Check sheet for the modelled part. Datum: model origin and axes. Units: mm. Round coordinates to 2 decimals unless told otherwise and drop trailing zeros. Write each loop counter-clockwise with the first axis right and the second up, starting at its lowest first coordinate (ties: lowest second). Pieces come first, ordered by that corner, then holes. Notation, with made-up numbers: (24.25, 79.5) -> (60.25, 79.5) arc R34 ccw to (60.25, 114.5) -> close; hole circle Ø5 at (60, 9). An arc over 180 degrees is marked (long way). Put each result on its own line as item: value. Start each with the question number.
from build123d import *

# Parameters (mm, degrees)
SKETCH1_R           = 4.7625
BOSS_EXTRUDE1_DEPTH = 4.7625


with BuildPart() as part:
    # Sketch1 → Boss-Extrude1 (new body)
    with BuildSketch(Plane.XY):
        Polygon((0, 0), (0, -45.252735849), (269.24, 127.295542021), (269.24, 172.54827787), align=None)
        with Locations(Location((9.525, -10.651818651, 0), (0, 0, 180))):
            Circle(SKETCH1_R, mode=Mode.SUBTRACT)
        with Locations(Location((28.575, -10.651818651, 0), (0, 0, 180))):
            Circle(SKETCH1_R, mode=Mode.SUBTRACT)
        with Locations(Location((239.234787134, 136.668181349, 0), (0, 0, 180))):
            Circle(SKETCH1_R, mode=Mode.SUBTRACT)
        with Locations(Location((258.284787134, 136.668181349, 0), (0, 0, 180))):
            Circle(SKETCH1_R, mode=Mode.SUBTRACT)
    extrude(amount=BOSS_EXTRUDE1_DEPTH)


solid = part.part
1. Gauge pin test, flat ends, axial feed: P1, Ø11, axis at x = 258.28, y = 136.67, coming from the -Z side; P2, Ø2, axis at y = 44, z = 2, coming from the +X side; P3, Ø1, axis at y = 110, z = 3.5, coming from the -X side. Record the tip position at first contact, or that the pin passes through.
2. Section check C-C, the plane x = 67. Enter the section's corners in (y, z), then the cut area to 3 significant figures.
3. Draft check along Y on faces 1 (the flat face through (136.5, 87.48, 2.35)), 2 (the flat face through (132.735, 39.814, 2.348)), 3 (the cylindrical face through (29.6, -6, 2.3)). Enter one of: released by +Y, released by -Y, zero draft, split by the parting line, or undercut.
4. Section check A-A, the plane z = 1.25. Enter the section's corners in (x, y) (1 decimal), then the cut area to 3 significant figures.
5. Section check B-B, the plane y = 46.5. Enter the section's corners in (x, z).
6. Material ranges on L1, parallel to X at y = -14, z = 2.2; L2, parallel to Y at x = 23, z = 0.5; L3, parallel to X at y = 102, z = 3.35, recorded low to high. Write a range as [from, to].
Reply:
1. P1: stops at z = 0
1. P2: stops at x = 140.83
1. P3: stops at x = 170.86
2. outline: (-2.31, 0) -> (42.94, 0) -> (42.94, 4.76) -> (-2.31, 4.76) -> close
2. area: 216 mm2
3. face 1: released by +Y
3. face 2: released by -Y
3. face 3: undercut
4. outline: (0, -45.3) -> (269.2, 127.3) -> (269.2, 172.5) -> (0, 0) -> close; hole circle Ø9.5 at (9.5, -10.7); hole circle Ø9.5 at (28.6, -10.7); hole circle Ø9.5 at (239.2, 136.7); hole circle Ø9.5 at (258.3, 136.7)
4. area: 11,900 mm2
5. outline: (72.56, 0) -> (143.17, 0) -> (143.17, 4.76) -> (72.56, 4.76) -> close
6. L1: x = [0, 6.14], [12.91, 25.19], [31.96, 48.77]
6. L2: y = [-30.51, 14.74]
6. L3: x = [159.16, 229.77]
